Check sheet for the modelled part. Datum: model origin and axes. Units: mm. A direction names the side the tool comes from. Give positions to 0.01 mm unless a question says otherwise; leave off trailing zeros. Write each loop counter-clockwise with the first axis right and the second up, starting at its lowest first coordinate (ties: lowest second). Pieces come first, ordered by that corner, then holes. Notation, with made-up numbers: (-2, 68) -> (16, 68) arc R16 cw to (16, 97) -> close; hole circle Ø2 at (86, 73.5). An arc over 180 degrees is marked (long way). Return JSON: item names as keys, results as strings.
from build123d import *

# Parameters (mm, degrees)
SKETCH1_R           = 35
BOSS_EXTRUDE1_DEPTH = 2
FILLET1_R           = 10
CUT_EXTRUDE2_REACH  = 51.538
SKETCH2_R           = 4.5
CUT_EXTRUDE3_REACH  = 51.538
SKETCH3_R           = 7.5
SKETCH3_R_2         = 7
BOSS_EXTRUDE2_DEPTH = 8


with BuildPart() as part:
    # Sketch1 → Boss-Extrude1 (new body)
    with BuildSketch(Plane.XY):
        Circle(SKETCH1_R)
        with BuildLine():
            Line((-10, 31.448370387), (-10, 5.773502692))
            Line((-10, 5.773502692), (-32.235087663, -7.063931156))
            ThreePointArc((-32.235087663, -7.063931156), (-28.578838325, 16.5), (-10, 31.448370387))
        make_face(mode=Mode.SUBTRACT)
        with BuildLine():
            Line((-22.235087663, -24.384439231), (0, -11.547005384))
            Line((0, -11.547005384), (22.235087663, -24.384439231))
            ThreePointArc((22.235087663, -24.384439231), (0, -33), (-22.235087663, -24.384439231))
        make_face(mode=Mode.SUBTRACT)
        with BuildLine():
            Line((32.235087663, -7.063931156), (10, 5.773502692))
            Line((10, 5.773502692), (10, 31.448370387))
            ThreePointArc((10, 31.448370387), (28.578838325, 16.5), (32.235087663, -7.063931156))
        make_face(mode=Mode.SUBTRACT)
    extrude(amount=BOSS_EXTRUDE1_DEPTH)

    # Fillet1
    fillet1_edges = [part.edges().sort_by_distance(p)[0] for p in [
        (-10, 5.773502692, 1),
        (10, 5.773502692, 1),
        (0, -11.547005384, 1),
    ]]
    fillet(fillet1_edges, radius=FILLET1_R)

    # Sketch2 → Cut-Extrude2 (cut, up to next)
    with BuildSketch(Plane(origin=(0, 0, 0), x_dir=(-1, 0, 0), z_dir=(0, 0, -1)), mode=Mode.PRIVATE) as cut_extrude2_sk1:
        Circle(SKETCH2_R)
    cut_extrude2_tool1 = extrude(cut_extrude2_sk1.sketch, amount=-CUT_EXTRUDE2_REACH, mode=Mode.PRIVATE) & part.part
    # Sketch2 → Cut-Extrude2 (cut, up to next)
    with BuildSketch(Plane(origin=(0, 0, 0), x_dir=(-1, 0, 0), z_dir=(0, 0, -1)), mode=Mode.PRIVATE) as cut_extrude2_sk2:
        with BuildLine():
            ThreePointArc((5, 0), (4.829629131, 1.294095226), (4.330127019, 2.5))
            Line((4.330127019, 2.5), (3.897114317, 2.25))
            ThreePointArc((3.897114317, 2.25), (4.346666218, 1.164685703), (4.5, 0))
            ThreePointArc((4.5, 0), (2.25, -3.897114317), (-2.25, -3.897114317))
            Line((-2.25, -3.897114317), (-2.5, -4.330127019))
            ThreePointArc((-2.5, -4.330127019), (2.5, -4.330127019), (5, 0))
        make_face()
    cut_extrude2_tool2 = extrude(cut_extrude2_sk2.sketch, amount=-CUT_EXTRUDE2_REACH, mode=Mode.PRIVATE) & part.part
    # Sketch2 → Cut-Extrude2 (cut, up to next)
    with BuildSketch(Plane(origin=(0, 0, 0), x_dir=(-1, 0, 0), z_dir=(0, 0, -1)), mode=Mode.PRIVATE) as cut_extrude2_sk3:
        with BuildLine():
            Line((2.25, 3.897114317), (2.5, 4.330127019))
            ThreePointArc((2.5, 4.330127019), (-3.535533906, 3.535533906), (-4.330127019, -2.5))
            Line((-4.330127019, -2.5), (-3.897114317, -2.25))
            ThreePointArc((-3.897114317, -2.25), (-3.181980515, 3.181980515), (2.25, 3.897114317))
        make_face()
    cut_extrude2_tool3 = extrude(cut_extrude2_sk3.sketch, amount=-CUT_EXTRUDE2_REACH, mode=Mode.PRIVATE) & part.part
    add(cut_extrude2_tool1.solids().sort_by_distance((0, 0, 0))[0], mode=Mode.SUBTRACT)
    add(cut_extrude2_tool2.solids().sort_by_distance((-2.446967, -4.238271, 0))[0], mode=Mode.SUBTRACT)
    add(cut_extrude2_tool3.solids().sort_by_distance((4.166654, -2.283144, 0))[0], mode=Mode.SUBTRACT)

    # Sketch3 → Cut-Extrude3 (cut, up to next)
    with BuildSketch(Plane(origin=(0, 0, 0), x_dir=(-1, 0, 0), z_dir=(0, 0, -1)), mode=Mode.PRIVATE) as cut_extrude3_sk1:
        with Locations((-12.990381057, -7.5)):
            Circle(SKETCH3_R)
    cut_extrude3_tool1 = extrude(cut_extrude3_sk1.sketch, amount=-CUT_EXTRUDE3_REACH, mode=Mode.PRIVATE) & part.part
    # Sketch3 → Cut-Extrude3 (cut, up to next)
    with BuildSketch(Plane(origin=(0, 0, 0), x_dir=(-1, 0, 0), z_dir=(0, 0, -1)), mode=Mode.PRIVATE) as cut_extrude3_sk2:
        with Locations((0, 17.5)):
            Circle(SKETCH3_R_2)
    cut_extrude3_tool2 = extrude(cut_extrude3_sk2.sketch, amount=-CUT_EXTRUDE3_REACH, mode=Mode.PRIVATE) & part.part
    add(cut_extrude3_tool1.solids().sort_by_distance((12.990381, -7.5, 0))[0], mode=Mode.SUBTRACT)
    add(cut_extrude3_tool2.solids().sort_by_distance((0, 17.5, 0))[0], mode=Mode.SUBTRACT)

    # Sketch3<4> → Boss-Extrude2 (add)
    with BuildSketch(Plane(origin=(0, 0, 0), x_dir=(-1, 0, 0), z_dir=(0, 0, -1))):
        with BuildLine():
            ThreePointArc((16.390381057, -7.5), (15.594932163, -9.685477873), (13.580784861, -10.84834636))
            Line((13.580784861, -10.84834636), (13.684973767, -11.439231012))
            ThreePointArc((13.684973767, -11.439231012), (16.054558829, -10.071150439), (16.990381057, -7.5))
            Line((16.990381057, -7.5), (16.390381057, -7.5))
        make_face()
        with BuildLine():
            Line((12.990381057, -3.5), (12.990381057, -4.1))
            ThreePointArc((12.990381057, -4.1), (15.17585893, -4.895448893), (16.338727417, -6.909596196))
            Line((16.338727417, -6.909596196), (16.929612069, -6.805407289))
            ThreePointArc((16.929612069, -6.805407289), (15.561531496, -4.435822228), (12.990381057, -3.5))
        make_face()
        with BuildLine():
            ThreePointArc((9.590381057, -7.5), (10.38582995, -5.314522127), (12.399977253, -4.15165364))
            Line((12.399977253, -4.15165364), (12.295788346, -3.560768988))
            ThreePointArc((12.295788346, -3.560768988), (9.926203284, -4.928849561), (8.990381057, -7.5))
            Line((8.990381057, -7.5), (9.590381057, -7.5))
        make_face()
        with BuildLine():
            ThreePointArc((12.990381057, -10.9), (10.804903184, -10.104551107), (9.642034697, -8.090403804))
            Line((9.642034697, -8.090403804), (9.051150045, -8.194592711))
            ThreePointArc((9.051150045, -8.194592711), (10.419230618, -10.564177772), (12.990381057, -11.5))
            Line((12.990381057, -11.5), (12.990381057, -10.9))
        make_face()
    extrude(amount=BOSS_EXTRUDE2_DEPTH)


solid = part.part
(1) Cross-section at B-B on z = -1.25. Enter the section's corners in (x, y), then the cut area to 3 significant figures.
Reply:
{"outline": "(-16.99, -7.5) arc R4 ccw to (-13.68, -11.44) -> (-13.58, -10.85) arc R3.4 cw to (-16.39, -7.5) -> close; (-16.93, -6.81) -> (-16.34, -6.91) arc R3.4 cw to (-12.99, -4.1) -> (-12.99, -3.5) arc R4 ccw to start; (-12.99, -11.5) arc R4 ccw to (-9.05, -8.19) -> (-9.64, -8.09) arc R3.4 cw to (-12.99, -10.9) -> close; (-12.4, -4.15) arc R3.4 cw to (-9.59, -7.5) -> (-8.99, -7.5) arc R4 ccw to (-12.3, -3.56) -> close", "area": "12.4 mm^2"}
(2) Cross-section at A-A on x = 0. Enter the section's corners in (y, z).
Reply:
{"outline": "(-35, 0) -> (-33, 0) -> (-33, 2) -> (-35, 2) -> close; (-13.09, 0) -> (-5, 0) -> (-5, 2) -> (-13.09, 2) -> close; (5, 0) -> (10.5, 0) -> (10.5, 2) -> (5, 2) -> close; (24.5, 0) -> (35, 0) -> (35, 2) -> (24.5, 2) -> close"}
(3) Set-up check for faces 5 (the cylindrical face through (-15.15, -4.874, -3.944)), 6 (the cylindrical face through (0.073, -13.094, 1.014)), 7 (the flat face through (-15.2, -4.7, -8)), 8 (the cylindrical face through (-16.03, -10.1, -3.94)): record each of +Z, -Z, +X, -X, +Y, -Y from which the full face is reachable in a straight line by a thin tool's end or side.
Reply:
{"face 5": "-Z", "face 6": "+Z, -Z", "face 7": "-Z, +X, -X, +Y, -Y", "face 8": "-Z, -X, -Y"}
(4) Thickness scan on L1, parallel to Y at x = 0, z = 0.95; L2, parallel to X at y = -3.5, z = 1.25; L3, parallel to Z at x = -11, y = 0. Record the ranges inside material, lowest first.
Reply:
{"L1": "-35 to -33, -13.09 to -5, 5 to 10.5, 24.5 to 35", "L2": "-34.82 to -32.81, -26.06 to -3.57, 2.83 to 6.65, 19.33 to 26.06, 32.81 to 34.82", "L3": "0 to 2"}
(5) Release check for a two-part mould opening along Y. For faces 1 (the flat face through (-10.2, -5.2, -8)), 2 (the cylindrical face through (-9.95, -4.9, -3.94)), 3 (the cylindrical face through (0, -33, 1)), 4 (the cylindrical face through (-3.194, 3.17, 0.986)) record: pulls with the +Y half, pulls with the -Y half, needs draft (parallel to the pull), parting line crosses it, or undercut.
Reply:
{"face 1": "needs draft", "face 2": "pulls with the +Y half", "face 3": "undercut", "face 4": "undercut"}
(6) Cross-section at D-D on x = -18.5. Enter the section's corners in (y, z), then the cut area to 3 significant figures.
Reply:
{"outline": "(-29.71, 0) -> (-27.33, 0) -> (-27.33, 2) -> (-29.71, 2) -> close; (-22.23, 0) -> (0.87, 0) -> (0.87, 2) -> (-22.23, 2) -> close; (27.33, 0) -> (29.71, 0) -> (29.71, 2) -> (27.33, 2) -> close", "area": "55.7 mm^2"}
(7) Cross-section at C-C on y = 25.5. Enter the section's corners in (x, z), then the cut area to 3 significant figures.
Reply:
{"outline": "(-23.97, 0) -> (-20.95, 0) -> (-20.95, 2) -> (-23.97, 2) -> close; (-10, 0) -> (10, 0) -> (10, 2) -> (-10, 2) -> close; (20.95, 0) -> (23.97, 0) -> (23.97, 2) -> (20.95, 2) -> close", "area": "52.1 mm^2"}
(8) Depth check by flat-ended pin: pin 1 Ø2 at (y, z) = (11.5, -2) entering from -X; pin 2 Ø6 at (y, z) = (-22, 0.5) entering from -X; pin 3 Ø1.6 at (y, z) = (20.5, 1.5) entering from +X; pin 4 Ø0.6 at (y, z) = (21.5, 1) entering from -X. Enter the tip coordinate at first touch or a pass-through.
Reply:
{"pin 1": "through", "pin 2": "x = -29.39", "pin 3": "x = 28.93", "pin 4": "x = -27.85"}
